from build123d import *

# Parameters (mm, degrees)
SKETCH_1_R          = 9.5
SKETCH_1_R_2        = 7
EXTRUDE_1_DEPTH     = 30
CHAMFER_1_SIZE      = 1
SKETCH_2_W          = 1
SKETCH_2_H          = 2
CUT_EXTRUDE_1_DEPTH = 33.870959828


with BuildPart() as part:
    # 스케치1 → 보스-돌출1 (new body)
    with BuildSketch(Plane.XY):
        Circle(SKETCH_1_R)
        Circle(SKETCH_1_R_2, mode=Mode.SUBTRACT)
    extrude(amount=EXTRUDE_1_DEPTH)

    # 모따기1
    chamfer_1_edges = [part.edges().sort_by_distance(p)[0] for p in [
        (-9.5, 0, 0),
        (-9.5, 0, 30),
    ]]
    chamfer(chamfer_1_edges, length=CHAMFER_1_SIZE)

    # 스케치2 → 컷-돌출1 (cut, through all)
    with BuildSketch(Plane.XY):
        Polygon((-3.633974596, 8.294228634), (-5.366025404, 7.294228634), (-5.866025404, 8.160254038), (-4.133974596, 9.160254038), align=None)
        with Locations((-9.5, 0)):
            Rectangle(SKETCH_2_W, SKETCH_2_H)
        Polygon((5.366025404, 7.294228634), (3.633974596, 8.294228634), (4.133974596, 9.160254038), (5.866025404, 8.160254038), align=None)
        with Locations((9.5, 0)):
            Rectangle(SKETCH_2_W, SKETCH_2_H)
        Polygon((3.633974596, -8.294228634), (5.366025404, -7.294228634), (5.866025404, -8.160254038), (4.133974596, -9.160254038), align=None)
        Polygon((-5.366025404, -7.294228634), (-3.633974596, -8.294228634), (-4.133974596, -9.160254038), (-5.866025404, -8.160254038), align=None)
    extrude(amount=CUT_EXTRUDE_1_DEPTH, mode=Mode.SUBTRACT)


solid = part.part
Build history of the part. All positions in model axes, mm. A direction names the side the tool comes from. Coordinates: 2 decimals unless noted, no trailing zeros. Write each loop counter-clockwise with the first axis right and the second up, starting at its lowest first coordinate (ties: lowest second). Pieces come first, ordered by that corner, then holes.
(1) Mould opens along X. For faces 1 (the cylindrical face through (8.255, 4.702, 14.804)), 2 (the cylindrical face through (-8.2, 4.8, 14.8)), 3 (the flat face through (-4.49, 7.8, 14.8)) say: pulls with the +X half, pulls with the -X half, needs draft (parallel to the pull), parting line crosses it, or undercut.
(2) Cut at C-C on z = 11.75. List the corners of the cut face in (x, y).
(3) Cut at A-A on y = 0. List the corners of the cut face in (x, z), and give its area (4 significant figures).
(4) Drill centre lines: line 1 (Y direction, x = 0, z = 15.25); line 2 (Y direction, x = -3, z = 9.5); line 3 (X direction, y = 0.75, z = 10). Where is each one in solid material? Low to high.
(5) Cut at B-B on x = 0. List the corners of the cut face in (y, z), and give its area (3 significant figures).
(6) 3-axis set-ups, long thin cutter, end or side, ignore diameter. For faces 4 (the cylindrical face through (6.466, -2.681, 14.79)), 5 (the flat face through (9, 0, 15)), 6 (the flat face through (-9, 0, 15)): which of +Z, -Z, +X, -X, +Y, -Y reach the whole face in a straight line?
(7) Pin check, flat tips, straight feed: pin 1 Ø0.5 at (x, z) = (-9, 16) entering from -Y; pin 2 Ø8.5 at (x, y) = (0, 0) entering from +Z; pin 3 Ø1 at (x, z) = (5.5, 8.5) entering from -Y; pin 4 Ø1.5 at (y, z) = (6, 22.5) entering from +X. Stop position of each tip, or through.
Working result:
1. face 1: pulls with the +X half
1. face 2: pulls with the -X half
1. face 3: undercut
2. outline: (-9.45, -1) arc R9.5 ccw to (-5.59, -7.68) - (-5.37, -7.29) - (-3.63, -8.29) - (-3.86, -8.68) arc R9.5 ccw to (3.86, -8.68) - (3.63, -8.29) - (5.37, -7.29) - (5.59, -7.68) arc R9.5 ccw to (9.45, -1) - (9, -1) - (9, 1) - (9.45, 1) arc R9.5 ccw to (5.59, 7.68) - (5.37, 7.29) - (3.63, 8.29) - (3.86, 8.68) arc R9.5 ccw to (-3.86, 8.68) - (-3.63, 8.29) - (-5.37, 7.29) - (-5.59, 7.68) arc R9.5 ccw to (-9.45, 1) - (-9, 1) - (-9, -1) - close; hole circle Ø14 at (0, 0)
3. outline: (-9, 0.5) - (-8.5, 0) - (-7, 0) - (-7, 30) - (-8.5, 30) - (-9, 29.5) - close; (7, 0) - (8.5, 0) - (9, 0.5) - (9, 29.5) - (8.5, 30) - (7, 30) - close
3. area: 119.5 mm2
4. line 1: y = -9.5 to -7, 7 to 9.5
4. line 2: y = -9.01 to -6.32, 6.32 to 9.01
4. line 3: x = -9 to -6.96, 6.96 to 9
5. outline: (-9.5, 1) - (-8.5, 0) - (-7, 0) - (-7, 30) - (-8.5, 30) - (-9.5, 29) - close; (7, 0) - (8.5, 0) - (9.5, 1) - (9.5, 29) - (8.5, 30) - (7, 30) - close
5. area: 148 mm2
6. face 4: +Z, -Z
6. face 5: +Z, -Z, +X
6. face 6: +Z, -Z, -X
7. pin 1: stops at y = -3.7
7. pin 2: passes through
7. pin 3: stops at y = -7.68
7. pin 4: stops at x = 7.92
